The listing builds one solid part. Answer for the finished solid, in the listing's coordinates (mm). Face numbers are marked on the shaded views. A direction names the side the tool comes from. Coordinates: 2 decimals unless noted, no trailing zeros. Loops run counter-clockwise (first coordinate to the right, second up) from the corner with the lowest first, then second, coordinate; pieces in that order, holes last. Notation, with made-up numbers: (12, 53) - (29, 53) arc R36 cw to (29, 92) - close; hole circle Ø2 at (53.25, -4). An arc over 180 degrees is marked (long way). Write each question's results on one line, items separated by ' | '. Start each with the question number.
(1) For the marked faces 1, 2 and 3, determine the directions among +Z, -Z, +X, -X, +Y, -Y from which every point of the face is accessible in a straight line to the end or side of a thin tool.
(2) Given pin 1 Ø8 at (x, y) = (-2, -156) entering from +Z; pin 2 Ø6 at (x, y) = (-1.5, -73) entering from -Z; pin 3 Ø1.5 at (x, y) = (5, -133) entering from +Z, each flat-ended and moving along its own axis, determine where each tip first touches the part or whether it passes through.
(3) Consider line 1 (Z direction, x = -0.5, y = -22); line 2 (X direction, y = -49.5, z = 4.5); line 3 (Z direction, x = -2.25, y = -71). Determine where each line is inside the solid, lowest interval first. Write a range as from..to.
(4) Find section B-B on y = 0. Determine the outline of the cut face in (x, z), then the cut area to 3 significant figures.
(5) Find section A-A on z = 0. Determine the outline of the cut face in (x, y), then the cut area to 3 significant figures.
(6) Find section D-D on y = -226.5. Determine the outline of the cut face in (x, z), then the cut area to 3 significant figures.
(7) Find section C-C on x = 0. Determine the outline of the cut face in (y, z).
from build123d import *

# Parameters (mm, degrees)
SKETCH1_W           = 15
SKETCH1_H           = 15
BOSS_EXTRUDE1_DEPTH = 7.5
SKETCH2_R           = 5
BOSS_EXTRUDE2_DEPTH = 50
SKETCH3_R           = 5
BOSS_EXTRUDE3_DEPTH = 300
FILLET1_R           = 1


with BuildPart() as part:
    # Sketch1 → Boss-Extrude1 (new body, symmetric)
    with BuildSketch(Plane(origin=(0, 0, 0), x_dir=(1, 0, 0), z_dir=(0, 1, 0))):
        Rectangle(SKETCH1_W, SKETCH1_H)
    extrude(amount=BOSS_EXTRUDE1_DEPTH, both=True)

    # Sketch2 → Boss-Extrude2 (add)
    with BuildSketch(Plane(origin=(0, 0, -7.5), x_dir=(-1, 0, 0), z_dir=(0, 0, -1))):
        Circle(SKETCH2_R)
    extrude(amount=BOSS_EXTRUDE2_DEPTH)

    # Sketch3 → Boss-Extrude3 (add)
    with BuildSketch(Plane.XZ.offset(7.5)):
        Circle(SKETCH3_R)
    extrude(amount=BOSS_EXTRUDE3_DEPTH)

    # Fillet1
    fillet1_edges = [part.edges().sort_by_distance(p)[0] for p in [
        (-7.5, 7.5, 0),
        (0, 7.5, 7.5),
        (-5, -7.5, 0),
        (7.5, 7.5, 0),
        (0, -7.5, 7.5),
        (-7.5, -7.5, 0),
        (0, -7.5, -7.5),
        (7.5, -7.5, 0),
        (0, 7.5, -7.5),
        (7.5, 0, 7.5),
        (-7.5, 0, 7.5),
        (-7.5, 0, -7.5),
        (7.5, 0, -7.5),
    ]]
    fillet(fillet1_edges, radius=FILLET1_R)


solid = part.part
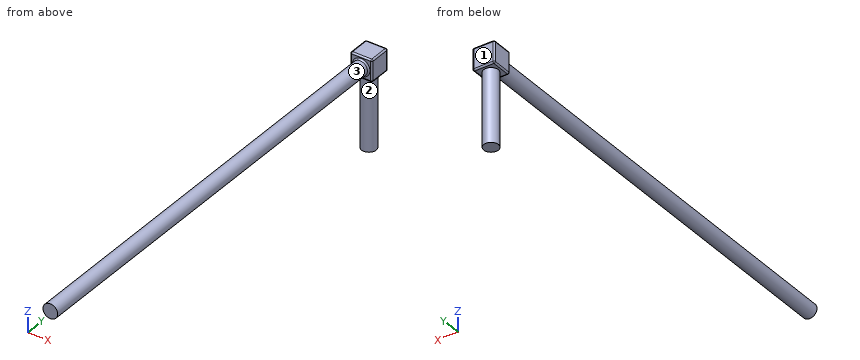
Values:
1) face 1: +Z, -Z, +X, -X, +Y | face 2: -Z | face 3: -Y
2) pin 1: stops at z = 5 | pin 2: stops at z = -5 | pin 3: stops at z = 2.63
3) line 1: z = -4.97..4.97 | line 2: x = -2.18..2.18 | line 3: z = -4.47..4.47
4) outline: (-7.5, -6.5) arc R1 ccw to (-6.5, -7.5) - (-5, -7.5) - (-5, -57.5) - (5, -57.5) - (5, -7.5) - (6.5, -7.5) arc R1 ccw to (7.5, -6.5) - (7.5, 6.5) arc R1 ccw to (6.5, 7.5) - (-6.5, 7.5) arc R1 ccw to (-7.5, 6.5) - close | area: 724 mm²
5) outline: (-7.5, -6.5) arc R1 ccw to (-6.5, -7.5) - (-6, -7.5) arc R1 cw to (-5, -8.5) - (-5, -307.5) - (5, -307.5) - (5, -8.5) arc R1 cw to (6, -7.5) - (6.5, -7.5) arc R1 ccw to (7.5, -6.5) - (7.5, 6.5) arc R1 ccw to (6.5, 7.5) - (-6.5, 7.5) arc R1 ccw to (-7.5, 6.5) - close | area: 3,220 mm²
6) outline: circle Ø10 at (0, 0) | area: 78.5 mm²
7) outline: (-307.5, -5) - (-8.5, -5) arc R1 cw to (-7.5, -6) - (-7.5, -6.5) arc R1 ccw to (-6.5, -7.5) - (-5, -7.5) - (-5, -57.5) - (5, -57.5) - (5, -7.5) - (6.5, -7.5) arc R1 ccw to (7.5, -6.5) - (7.5, 6.5) arc R1 ccw to (6.5, 7.5) - (-6.5, 7.5) arc R1 ccw to (-7.5, 6.5) - (-7.5, 6) arc R1 cw to (-8.5, 5) - (-307.5, 5) - close
